Check sheet for the modelled part. Datum: model origin and axes. Units: mm. A direction names the side the tool comes from. Give positions to 0.01 mm unless a question says otherwise; leave off trailing zeros. Write each loop counter-clockwise with the first axis right and the second up, starting at its lowest first coordinate (ties: lowest second). Pieces come first, ordered by that corner, then holes. Notation, with made-up numbers: (-12.5, -4.5) -> (37.5, -4.5) arc R20 cw to (37.5, 17.5) -> close; hole circle Ø9 at (25, 65). An arc over 180 degrees is marked (long way). Answer as a JSON object with one key per item and string values.
from build123d import *

# Parameters (mm, degrees)
SKETCH1_R                 = 31.75
CENTERCIRCLEEXTRUDE_DEPTH = 19.558
SKETCH2_R                 = 80.01
BASEEXPAND_DEPTH          = 7.62
FILLET15_R                = 3.175
SKETCH3_R                 = 27.559
CENTERCUT_DEPTH           = 27.178
SKETCH4_R                 = 6.731
OUTERCIRCLECUT_DEPTH      = 7.62
SKETCH8_R                 = 80.01
STARFISHCUT_DEPTH         = 7.62
BATMAN_CUT_DEPTH          = 5.08
FILLET12_R                = 6.35


with BuildPart() as part:
    # Sketch1 → CenterCircleExtrude (new body)
    with BuildSketch(Plane(origin=(0, 0, 0), x_dir=(1, 0, 0), z_dir=(0, 1, 0))):
        with Locations(Location((0, 0, 0), (0, 0, 270))):
            Circle(SKETCH1_R)
    extrude(amount=CENTERCIRCLEEXTRUDE_DEPTH)

    # Sketch2 → BaseExpand (add)
    with BuildSketch(Plane.XZ):
        with Locations(Location((0, 0, 0), (0, 0, 90))):
            Circle(SKETCH2_R)
    extrude(amount=BASEEXPAND_DEPTH)

    # Fillet15
    fillet15_edges = [part.edges().sort_by_distance(p)[0] for p in [
        (0, 0, -31.75),
    ]]
    fillet(fillet15_edges, radius=FILLET15_R)

    # Sketch3 → CenterCut (cut)
    with BuildSketch(Plane(origin=(0, 19.558, 0), x_dir=(1, 0, 0), z_dir=(0, 1, 0))):
        with Locations(Location((0, 0, 0), (0, 0, 270))):
            Circle(SKETCH3_R)
    extrude(amount=-CENTERCUT_DEPTH, mode=Mode.SUBTRACT)

    # Sketch4 → OuterCircleCut (cut)
    with BuildSketch(Plane(origin=(0, 0, 0), x_dir=(1, 0, 0), z_dir=(0, 1, 0))):
        with Locations(Location((0, 55.118, 0), (0, 0, 270))):
            Circle(SKETCH4_R)
        with Locations(Location((52.420333065, 17.032398696, 0), (0, 0, 270))):
            Circle(SKETCH4_R)
        with Locations(Location((32.397547536, -44.591398696, 0), (0, 0, 270))):
            Circle(SKETCH4_R)
        with Locations(Location((-32.397547536, -44.591398696, 0), (0, 0, 270))):
            Circle(SKETCH4_R)
        with Locations(Location((-52.420333065, 17.032398696, 0), (0, 0, 270))):
            Circle(SKETCH4_R)
    extrude(amount=-OUTERCIRCLECUT_DEPTH, mode=Mode.SUBTRACT)

    # Sketch8 → StarfishCut (cut)
    with BuildSketch(Plane(origin=(0, 0, 0), x_dir=(1, 0, 0), z_dir=(0, 1, 0))):
        Circle(SKETCH8_R)
        with BuildLine():
            ThreePointArc((-60.451485692, 10.809361858), (-62.083067271, 20.172011359), (-55.259862746, 26.787534327))
            ThreePointArc((-55.259862746, 26.787534327), (-52.990125634, 27.176408575), (-50.691117004, 27.044162367))
            ThreePointArc((-50.691117004, 27.044162367), (-36.498445494, 28.482280038), (-22.436174146, 30.88074446))
            ThreePointArc((-22.436174146, 30.88074446), (-15.809618103, 43.513592992), (-10.056110229, 56.567222915))
            ThreePointArc((-10.056110229, 56.567222915), (-9.47145111, 58.794576379), (-8.400222382, 60.833055899))
            ThreePointArc((-8.400222382, 60.833055899), (0, 65.278), (8.400222382, 60.833055899))
            ThreePointArc((8.400222382, 60.833055899), (9.47145111, 58.794576379), (10.056110229, 56.567222915))
            ThreePointArc((10.056110229, 56.567222915), (15.809618103, 43.513592992), (22.436174146, 30.88074446))
            ThreePointArc((22.436174146, 30.88074446), (36.498445494, 28.482280038), (50.691117004, 27.044162367))
            ThreePointArc((50.691117004, 27.044162367), (52.990125634, 27.176408575), (55.259862746, 26.787534327))
            ThreePointArc((55.259862746, 26.787534327), (60.546685924, 23.130594267), (62.580333065, 17.032398696))
            ThreePointArc((62.580333065, 17.032398696), (62.033399971, 13.743851196), (60.451485692, 10.809361858))
            ThreePointArc((60.451485692, 10.809361858), (58.843804343, 9.160637981), (56.90613492, 7.916304043))
            ThreePointArc((56.90613492, 7.916304043), (46.26932683, -1.589400596), (36.302492346, -11.795394786))
            ThreePointArc((36.302492346, -11.795394786), (38.366897955, -25.910575851), (41.384943465, -39.853011375))
            ThreePointArc((41.384943465, -39.853011375), (42.22114982, -41.998632188), (42.552695773, -44.27744921))
            ThreePointArc((42.552695773, -44.27744921), (42.556334523, -44.434405209), (42.557547536, -44.591398696))
            ThreePointArc((42.557547536, -44.591398696), (38.241722309, -52.902308467), (28.960850446, -54.152502874))
            ThreePointArc((28.960850446, -54.152502874), (26.896020001, -53.132990748), (25.11381532, -51.674677951))
            ThreePointArc((25.11381532, -51.674677951), (12.786398515, -44.495896582), (0, -38.170699348))
            ThreePointArc((0, -38.170699348), (-12.786398515, -44.495896582), (-25.11381532, -51.674677951))
            ThreePointArc((-25.11381532, -51.674677951), (-26.896020001, -53.132990748), (-28.960850446, -54.152502874))
            ThreePointArc((-28.960850446, -54.152502874), (-38.369445699, -52.811011359), (-42.552695773, -44.27744921))
            ThreePointArc((-42.552695773, -44.27744921), (-42.22114982, -41.998632188), (-41.384943465, -39.853011375))
            ThreePointArc((-41.384943465, -39.853011375), (-38.366897955, -25.910575851), (-36.302492346, -11.795394786))
            ThreePointArc((-36.302492346, -11.795394786), (-46.26932683, -1.589400596), (-56.90613492, 7.916304043))
            ThreePointArc((-56.90613492, 7.916304043), (-58.843804343, 9.160637981), (-60.451485692, 10.809361858))
        make_face(mode=Mode.SUBTRACT)
    extrude(amount=-STARFISHCUT_DEPTH, mode=Mode.SUBTRACT)

    # Sketch14 → Batman Cut (cut)
    with BuildSketch(Plane(origin=(0, 0, 0), x_dir=(1, 0, 0), z_dir=(0, 1, 0))):
        with BuildLine():
            Line((-29.28146985, -22.804327102), (-12.639732086, -34.895257327))
            ThreePointArc((-12.639732086, -34.895257327), (-11.563303962, -41.691557027), (-18.359603662, -42.767985152))
            Line((-18.359603662, -42.767985152), (-35.001341426, -30.677054926))
            ThreePointArc((-35.001341426, -30.677054926), (-36.07776955, -23.880755226), (-29.28146985, -22.804327102))
        make_face()
        with BuildLine():
            Line((-30.736675694, 20.801408088), (-37.093253888, 1.237872028))
            ThreePointArc((-37.093253888, 1.237872028), (-43.224284421, -1.88604406), (-46.348200509, 4.244986472))
            Line((-46.348200509, 4.244986472), (-39.991622315, 23.808522532))
            ThreePointArc((-39.991622315, 23.808522532), (-33.860591782, 26.93243862), (-30.736675694, 20.801408088))
        make_face()
        with BuildLine():
            Line((10.28515957, 35.660304314), (-10.28515957, 35.660304314))
            ThreePointArc((-10.28515957, 35.660304314), (-15.150772949, 40.525917694), (-10.28515957, 45.391531073))
            Line((-10.28515957, 45.391531073), (10.28515957, 45.391531073))
            ThreePointArc((10.28515957, 45.391531073), (15.150772949, 40.525917694), (10.28515957, 35.660304314))
        make_face()
        with BuildLine():
            Line((37.093253888, 1.237872028), (30.736675694, 20.801408088))
            ThreePointArc((30.736675694, 20.801408088), (33.860591782, 26.93243862), (39.991622315, 23.808522532))
            Line((39.991622315, 23.808522532), (46.348200509, 4.244986472))
            ThreePointArc((46.348200509, 4.244986472), (43.224284421, -1.88604406), (37.093253888, 1.237872028))
        make_face()
        with BuildLine():
            Line((12.639732086, -34.895257327), (29.28146985, -22.804327102))
            ThreePointArc((29.28146985, -22.804327102), (36.07776955, -23.880755226), (35.001341426, -30.677054926))
            Line((35.001341426, -30.677054926), (18.359603662, -42.767985152))
            ThreePointArc((18.359603662, -42.767985152), (11.563303962, -41.691557027), (12.639732086, -34.895257327))
        make_face()
    extrude(amount=-BATMAN_CUT_DEPTH, mode=Mode.SUBTRACT)

    # Fillet12
    fillet12_edges = [part.edges().sort_by_distance(p)[0] for p in [
        (-22.436174146, -3.81, -30.88074446),
        (-36.302492346, -3.81, 11.795394786),
        (0, -3.81, 38.170699348),
        (36.302492346, -3.81, 11.795394786),
        (22.436174146, -3.81, -30.88074446),
    ]]
    fillet(fillet12_edges, radius=FILLET12_R)


solid = part.part
1. Sectioned sample at A-A, the plane y = 17.25. Enter the section's corners in (x, z), plus the area to 3 significant figures.
Determined:
{"outline": "circle Ø63.5 at (0, 0); hole circle Ø55.12 at (0, 0)", "area": "781 mm^2"}
2. Sectioned sample at C-C, the plane z = -41. Enter the section's corners in (x, y), plus the area to 3 significant figures.
Determined:
{"outline": "(-17.04, -7.62) -> (17.04, -7.62) -> (17.04, 0) -> (15.13, 0) -> (15.13, -5.08) -> (-15.13, -5.08) -> (-15.13, 0) -> (-17.04, 0) -> close", "area": "106 mm^2"}
3. Sectioned sample at B-B, the plane x = 0. State how many separate pieces and enclosed holes the cut face has, plus the area to 3 significant figures.
Determined:
{"separate pieces": "3", "enclosed holes": "0", "area": "389 mm^2"}
4. Mould release check, pull along X, two halves, no side actions. Record for faces 4 (the face through (26, 19.558, -10)), 5 (the face through (43.33, -2.5, 1.85)), 6 (the face through (-30.995, 11.252, -6.883)): released by +X, released by -X, zero draft, split by the parting line, or undercut.
Determined:
{"face 4": "zero draft", "face 5": "undercut", "face 6": "split by the parting line"}
5. Access from +Z, -Z, +X, -X, +Y, -Y to the whole of each face (thin tool, end or side, straight path). Record for faces 1 (the face through (-33.87, -2.5, -11.16)), 2 (the face through (38.604, -3.757, 27.198)), 3 (the face through (-38.67, -3.76, 27.55)).
Determined:
{"face 1": "+Y", "face 2": "+X, +Y, -Y", "face 3": "-X, +Y, -Y"}
6. Scan lines: L1, parallel to Y at x = 30.5, z = 37.5; L2, parallel to Y at x = 0, z = -43; L3, parallel to X at y = 15.5, z = -3.5. Record each from-to range of solid material in increasing order. Write a range as [from, to].
Determined:
{"L1": "[-7.62, 0]", "L2": "[-7.62, -5.08]", "L3": "[-31.56, -27.34], [27.34, 31.56]"}
7. Go/stop test with flat-tipped pins: P1, Ø17.5, axis at x = -32.4, z = 44.59, coming from the +Y side; P2, Ø17.5, axis at x = -38, z = -19, coming from the +Y side; P3, Ø1.5, axis at x = 1, y = -2, coming from the +Z side; P4, Ø11, axis at x = 32.4, z = 44.59, coming from the +Y side. Record where each tip stops, or that it passes through.
Determined:
{"P1": "y = 0", "P2": "y = 0.23", "P3": "z = 39.06", "P4": "through"}
